```python
from build123d import *

# Parameters (mm, degrees)
F0_W           = 118.999
F0_H           = 119
F1_DEPTH       = 12.7
F3_D           = 8.255
F3_CBORE_D     = 14.5
F3_CBORE_DEPTH = 9.525
F5_D           = 6.8


with BuildPart() as f1:
    # F0 (on Top) → F1 (new body, symmetric)
    with BuildSketch(Plane.XY):
        Rectangle(F0_W, F0_H)
    extrude(amount=F1_DEPTH, both=True)

    # F3 (through all)
    with Locations(Plane.XY.offset(12.7)):
        with Locations((-37.1149003506, -37.5026), (-37.4969, 37.5036), (37.5031, 37.5036), (37.8850996494, -37.4964)):
            CounterBoreHole(F3_D / 2, F3_CBORE_D / 2, F3_CBORE_DEPTH)

    # F5 (through all)
    with Locations(Plane.XY.offset(12.7)):
        with Locations((0, 0)):
            Hole(F5_D / 2)


solid = f1.part
```
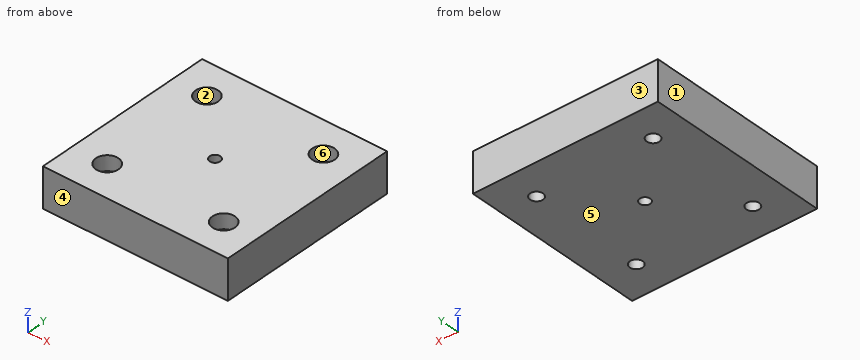
Geometry check sheet. Reference: the model listing, model coordinates, mm. Face numbers are marked on the shaded views. A direction names the side the tool comes from. Round coordinates to 2 decimals unless told otherwise and drop trailing zeros. Order: outer loops, then holes, each group sorted by start corner. A loop starts at its lowest first (then second) coordinate and runs counter-clockwise, first axis right, second up. Notation, with made-up numbers: (25, 65.5) - (37, 65.5) arc R19 cw to (37, 72.5) - close; hole circle Ø2 at (26, 1.5). An arc over 180 degrees is marked (long way). Use a Markdown table: item, result. Add a question column.
1) Section check A-A (y = 0). Record the cut outline in (x, z), then the cut area to 3 significant figures.
2) Mould release check, pull along Y, two halves, no side actions. Record for the marked faces 1, 2, 3 and 4: released by +Y, released by -Y, zero draft, split by the parting line, or undercut.
3) Gauge pin test, flat end, axial feed: P1, Ø10.5, axis at x = 37.5, y = 37.5, coming from the +Z side (3 decimals). Record the tip position at first contact, or that the pin passes through.
4) Section check C-C (x = 39.5). Record the cut outline in (y, z) (3 decimals), then the cut area to 3 significant figures.
5) Set-up check for the marked faces 5 and 6: record each of +Z, -Z, +X, -X, +Y, -Y from which the full face is reachable in a straight line by a thin tool's end or side.
6) Thickness scan on line 1 along X through (y, z) = (-35.5, -8.25); line 2 along X through (y, z) = (39, -4.5); line 3 along Y through (x, z) = (-2, -4.75). Record the ranges inside material, lowest first.
7) Section check D-D (z = -11). Record the cut outline in (x, y) (1 decimal), then the cut area to 3 significant figures.
Established:
| question | item | result |
|---|---|---|
| 1 | outline | (-59.5, -12.7) - (-3.4, -12.7) - (-3.4, 12.7) - (-59.5, 12.7) - close; (3.4, -12.7) - (59.5, -12.7) - (59.5, 12.7) - (3.4, 12.7) - close |
| 1 | area | 2,850 mm2 |
| 2 | face 1 | zero draft |
| 2 | face 2 | undercut |
| 2 | face 3 | released by +Y |
| 2 | face 4 | released by -Y |
| 3 | P1 | z = 3.175 |
| 4 | outline | (-59.5, -12.7) - (-41.295, -12.7) - (-41.295, 3.175) - (-44.564, 3.175) - (-44.564, 12.7) - (-59.5, 12.7) - close; (-33.698, -12.7) - (33.891, -12.7) - (33.891, 3.175) - (30.534, 3.175) - (30.534, 12.7) - (-30.429, 12.7) - (-30.429, 3.175) - (-33.698, 3.175) - close; (41.116, -12.7) - (59.5, -12.7) - (59.5, 12.7) - (44.473, 12.7) - (44.473, 3.175) - (41.116, 3.175) - close |
| 4 | area | 2,520 mm2 |
| 5 | face 5 | -Z, +X, -X, +Y, -Y |
| 5 | face 6 | +Z |
| 6 | line 1 | -59.5 to -40.72, -33.51 to 34.27, 41.5 to 59.5 |
| 6 | line 2 | -59.5 to -41.34, -33.65 to 33.66, 41.35 to 59.5 |
| 6 | line 3 | -59.5 to -2.75, 2.75 to 59.5 |
| 7 | outline | (-59.5, -59.5) - (59.5, -59.5) - (59.5, 59.5) - (-59.5, 59.5) - close; hole circle Ø8.3 at (-37.5, 37.5); hole circle Ø8.3 at (-37.1, -37.5); hole circle Ø6.8 at (0, 0); hole circle Ø8.3 at (37.5, 37.5); hole circle Ø8.3 at (37.9, -37.5) |
| 7 | area | 13,900 mm2 |
